Design review of the part built by this model. Coordinates are the model's own, in mm. Face numbers are marked on the shaded views. A direction names the side the tool comes from. Give positions to 0.01 mm unless a question says otherwise; leave off trailing zeros. Write each loop counter-clockwise with the first axis right and the second up, starting at its lowest first coordinate (ties: lowest second). Pieces come first, ordered by that corner, then holes. Notation, with made-up numbers: (-39, 18) -> (6, 18) arc R21 ccw to (6, 24) -> close; hole circle Ø2 at (4.25, 73.25). An arc over 180 degrees is marked (long way). Use CSV: the item, a comma, the result in double quotes.
```python
from build123d import *

# Parameters (mm, degrees)
F0_R     = 10.541
F1_DEPTH = 0.8128
F2_R     = 4.1275
F3_DEPTH = 8.89
F5_R     = 10.541
F6_DEPTH = 0.8128
F7_R     = 3.1115
F8_DEPTH = 8.89
F9_SIZE  = 2.54


with BuildPart() as f1:
    # F0 (on Top) → F1 (new body)
    with BuildSketch(Plane.XY):
        Circle(F0_R)
    extrude(amount=F1_DEPTH)

    # F2 (on Top) → F3 (join)
    with BuildSketch(Plane.XY):
        Circle(F2_R)
    extrude(amount=F3_DEPTH)

    # F5 (on offset) → F6 (join)
    with BuildSketch(Plane.XY.offset(8.89)):
        Circle(F5_R)
    extrude(amount=-F6_DEPTH)

    # F7 (on Top) → F8 (cut)
    with BuildSketch(Plane.XY):
        Circle(F7_R)
    extrude(amount=F8_DEPTH, mode=Mode.SUBTRACT)

    # F9
    f9_edges = [f1.edges().sort_by_distance(p)[0] for p in [
        (-4.1275, 0, 8.0772),
        (-4.1275, 0, 0.8128),
    ]]
    chamfer(f9_edges, length=F9_SIZE)


solid = f1.part
```
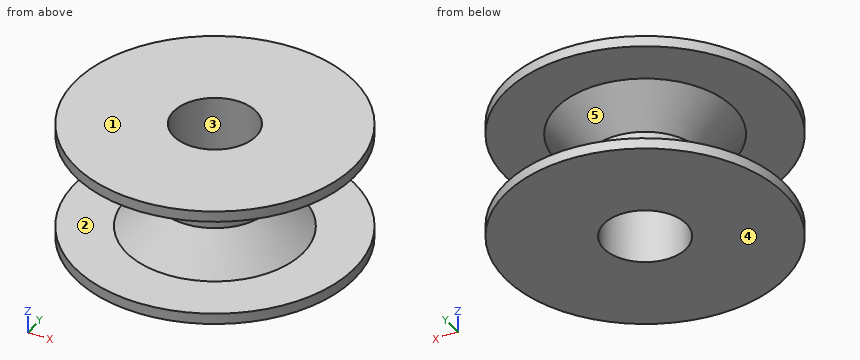
(1) Take a section at C-C (y = 7.5). Write out the cut boundary in (x, z).
Established:
outline,"(-7.41, 0) -> (7.41, 0) -> (7.41, 0.81) -> (-7.41, 0.81) -> close; (-7.41, 8.08) -> (7.41, 8.08) -> (7.41, 8.89) -> (-7.41, 8.89) -> close"
(2) Take a section at D-D (z = 7.5). Write out the cut boundary in (x, y).
Established:
outline,"circle Ø12.18 at (0, 0); hole circle Ø6.22 at (0, 0)"
(3) For line 1 along Z through (x, y) = (-5.75, -5.75); line 2 along Y through (x, z) = (0, 5.5); line 3 along Y through (x, z) = (2.5, 1), list the stretches that pass through material, from the lowest coordinate up. Write a range as [from, to].
Established:
line 1,"z = [0, 0.81], [8.08, 8.89]"
line 2,"y = [-4.13, -3.11], [3.11, 4.13]"
line 3,"y = [-5.98, -1.85], [1.85, 5.98]"
(4) Mouldability with a two-part tool opening along X and no side actions: class the marked faces 3, 4 and 5 as +X half, -X half, draft (parallel to the pull), parting line (faces both ways), or undercut.
Established:
face 3,"undercut"
face 4,"draft"
face 5,"parting line"
(5) Tool access review of the marked faces 1 and 2: name each direction out of +Z, -Z, +X, -X, +Y, -Y from which nothing blocks a thin tool from reaching the whole face with its end or side.
Established:
face 1,"+Z, +X, -X, +Y, -Y"
face 2,"none"
(6) Take a section at A-A (y = 0). Write out the cut boundary in (x, z).
Established:
outline,"(-10.54, 0) -> (-3.11, 0) -> (-3.11, 8.89) -> (-10.54, 8.89) -> (-10.54, 8.08) -> (-6.67, 8.08) -> (-4.13, 5.54) -> (-4.13, 3.35) -> (-6.67, 0.81) -> (-10.54, 0.81) -> close; (3.11, 0) -> (10.54, 0) -> (10.54, 0.81) -> (6.67, 0.81) -> (4.13, 3.35) -> (4.13, 5.54) -> (6.67, 8.08) -> (10.54, 8.08) -> (10.54, 8.89) -> (3.11, 8.89) -> close"
(7) Clearance check with flat-ended pins moving along their axes: pin 1 (12 mm diameter, centred on x = 7.5, y = -7.5, fed in from -Z); pin 2 (1.5 mm diameter, centred on y = -1.5, z = 6, fed in from +X); pin 3 (1 mm diameter, centred on y = 2, z = 2, fed in from +X); pin 4 (3 mm diameter, centred on x = -6.5, z = 7.5, fed in from +Y). State where each tip first meets the part, or that it passes through.
Established:
pin 1,"stops at z = 0"
pin 2,"stops at x = 5.15"
pin 3,"stops at x = 5.66"
pin 4,"stops at y = 9.22"
